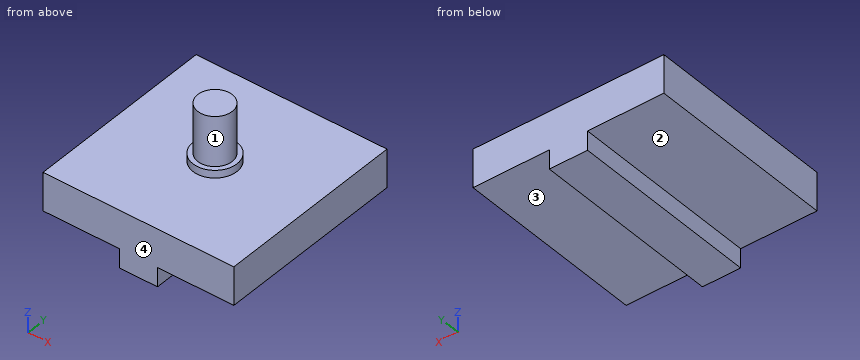
Autodesk Inventor part; units mm, degrees
ref_plane "YZ Plane" through (0, 0, 0) normal (1, 0, 0) x (0, 1, 0)
ref_plane "XZ Plane" through (0, 0, 0) normal (0, 1, 0) x (-1, 0, 0)
ref_plane "XY Plane" through (0, 0, 0) normal (0, 0, 1) x (1, 0, 0)
sketch "Sketch1" plane through (0, 0, 0) normal (0, 0, 1) x (1, 0, 0)
  line L0 (-5, -5) -> (5, -5)
  line L1 (5, -5) -> (5, 5)
  line L2 (5, 5) -> (-5, 5)
  line L3 (-5, 5) -> (-5, -5)
  line L4 (-5, -5) -> (5, 5) construction
  line L5 (5, -5) -> (-5, 5) construction
  point P0 (0, 0)
  dimension "d0" = 10
  dimension "d1" = 10
extrude "Extrusion1" add sketch "Sketch1" along normal blind 2
sketch "Sketch2" plane through (0, 0, 2) normal (0, 0, 1) x (1, 0, 0)
  circle A0 centre (0, 0) radius 0.9
  dimension "d4" = 1.8
extrude "Extrusion2" add sketch "Sketch2" along normal blind 3
sketch "Sketch4" plane through (0, 0, 0) normal (0, 0, -1) x (-1, 0, 0)
  line L0 (5, -5) -> (-5, -5)
  line L1 (1, 5) -> (-1, 5)
  line L2 (-1, 5) -> (-1, -5)
  line L3 (-1, -5) -> (1, -5)
  line L4 (1, -5) -> (1, 5)
  circle A0 centre (0, 0) radius 0.9
  line L5 (1, 5) -> (-1, -5) construction
  line L6 (-1, 5) -> (1, -5) construction
  dimension "d7" = 2
extrude "Extrusion3" add sketch "Sketch4" along normal blind 1 contours L0 L2 L1 L4 | A0
sketch "Sketch5" plane through (0, 0, 2) normal (0, 0, 1) x (1, 0, 0)
  circle A0 centre (0, 0) radius 0.9
  circle A1 centre (0, 0) radius 1.15
  dimension "d10" = 2.3
extrude "Extrusion4" add sketch "Sketch5" along normal blind 0.4
properties part number "TrzymakNaLozysko"
The model under review builds one solid part; all positions refer to its coordinate system, in mm. Face numbers are marked on the shaded views. A direction names the side the tool comes from. Round coordinates to 2 decimals unless told otherwise and drop trailing zeros. Order: outer loops, then holes, each group sorted by start corner. A loop starts at its lowest first (then second) coordinate and runs counter-clockwise, first axis right, second up. Notation, with made-up numbers: (15.5, 40.5) -> (43.5, 40.5) arc R21 cw to (43.5, 73.5) -> close; hole circle Ø8 at (-3.75, -8.75). An arc over 180 degrees is marked (long way). Return JSON: item names as keys, results as strings.
1. Insertion check: P1, Ø2, axis at x = -3.5, z = 4, coming from the +Y side; P2, Ø1, axis at x = 2, y = -1, coming from the +Z side; P3, Ø0.8, axis at y = 2.5, z = -0.5, coming from the -X side; P4, Ø0.5, axis at y = -2, z = -0.5, coming from the +X side. Each pin has a flat end and moves straight along its axis. Give the tip position at first contact, or say it passes through.
Answer block:
{"P1": "passes through", "P2": "stops at z = 2", "P3": "stops at x = -1", "P4": "stops at x = 1"}
2. For L1, parallel to Z at x = -3.5, y = 3; L2, parallel to Z at x = 0, y = -4.5; L3, parallel to X at y = 4.25, z = -0.2, list the stretches that pass through material, from the lowest coordinate up. Write a range as [from, to].
Answer block:
{"L1": "z = [0, 2]", "L2": "z = [-1, 2]", "L3": "x = [-1, 1]"}
3. For the marked faces 1, 2, 3 and 4, list the 3-axis set-ups (+Z, -Z, +X, -X, +Y, -Y) from which the entire face can be reached by the end or side of a thin tool; tool diameter is ignored.
Answer block:
{"face 1": "+Z", "face 2": "-Z, -X, +Y, -Y", "face 3": "-Z, +X, +Y, -Y", "face 4": "+Z, -Z, +X, -X, -Y"}
4. Take a section at D-D (x = -4). Write out the cut boundary in (y, z), then the cut area to 3 significant figures.
Answer block:
{"outline": "(-5, 0) -> (5, 0) -> (5, 2) -> (-5, 2) -> close", "area": "20.0 mm²"}
5. Take a section at B-B (x = 0). Write out the cut boundary in (y, z), then the cut area to 3 significant figures.
Answer block:
{"outline": "(-5, -1) -> (5, -1) -> (5, 2) -> (1.15, 2) -> (1.15, 2.4) -> (0.9, 2.4) -> (0.9, 5) -> (-0.9, 5) -> (-0.9, 2.4) -> (-1.15, 2.4) -> (-1.15, 2) -> (-5, 2) -> close", "area": "35.6 mm²"}
6. Take a section at A-A (y = 4.25). Write out the cut boundary in (x, z).
Answer block:
{"outline": "(-5, 0) -> (-1, 0) -> (-1, -1) -> (1, -1) -> (1, 0) -> (5, 0) -> (5, 2) -> (-5, 2) -> close"}
7. Take a section at C-C (y = 0). Write out the cut boundary in (x, z).
Answer block:
{"outline": "(-5, 0) -> (-1, 0) -> (-1, -1) -> (1, -1) -> (1, 0) -> (5, 0) -> (5, 2) -> (1.15, 2) -> (1.15, 2.4) -> (0.9, 2.4) -> (0.9, 5) -> (-0.9, 5) -> (-0.9, 2.4) -> (-1.15, 2.4) -> (-1.15, 2) -> (-5, 2) -> close"}
